```python
from build123d import *

# Parameters (mm, degrees)
F1_DEPTH = 150.876
F2_R     = 5.08


with BuildPart() as f1:
    # F0 (on Front) → F1 (new body)
    with BuildSketch(Plane.XZ):
        with BuildLine():
            Line((0, 22.650681), (0, 0))
            Line((0, 0), (53.119011, 0))
            Line((53.119011, 0), (53.119011, 22.650681))
            ThreePointArc((53.119011, 22.650681), (51.259139, 27.140809), (46.769011, 29.000681))
            Line((46.769011, 29.000681), (6.35, 29.000681))
            ThreePointArc((6.35, 29.000681), (1.859872, 27.140809), (0, 22.650681))
        make_face()
    extrude(amount=F1_DEPTH)

    # F2
    f2_edges = [f1.edges().sort_by_distance(p)[0] for p in [
        (53.119011, -75.438, 0),
        (26.559506, -150.876, 0),
        (0, -75.438, 0),
        (26.559506, 0, 0),
    ]]
    fillet(f2_edges, radius=F2_R)


solid = f1.part
```
Model file for the job. Use its own axes, mm. Round coordinates to 2 decimals unless told otherwise and drop trailing zeros. Write each loop counter-clockwise with the first axis right and the second up, starting at its lowest first coordinate (ties: lowest second). Pieces come first, ordered by that corner, then holes. Notation, with made-up numbers: (83, 62) -> (125, 62) arc R13 cw to (125, 86) -> close; hole circle Ø6 at (1.25, 27). An arc over 180 degrees is marked (long way). Answer as CSV lines item,"result".
1. Pin check, flat tip, straight feed: pin 1 Ø3 at (y, z) = (-32, 25.5) entering from +X. Stop position of the tip, or through.
Resolved:
pin 1,"x = 52.97"
2. Drill centre lines: line 1 (X direction, y = -130, z = 4.5); line 2 (Z direction, x = 6, y = -65); line 3 (X direction, y = -85.5, z = 25.25). Where is each one in solid material? Low to high.
Resolved:
line 1,"0.03 to 53.09"
line 2,"0 to 28.99"
line 3,"0.56 to 52.56"
3. Slice it at A-A, the plane y = -97. List the corners of the cut face in (x, z).
Resolved:
outline,"(0, 5.08) arc R5.08 ccw to (5.08, 0) -> (48.04, 0) arc R5.08 ccw to (53.12, 5.08) -> (53.12, 22.65) arc R6.35 ccw to (46.77, 29) -> (6.35, 29) arc R6.35 ccw to (0, 22.65) -> close"
